Read the model definition and answer for the solid it produces. Units are mm, in the model's axes. A direction names the side the tool comes from. Round coordinates to 2 decimals unless told otherwise and drop trailing zeros. Loops run counter-clockwise (first coordinate to the right, second up) from the corner with the lowest first, then second, coordinate; pieces in that order, holes last. Notation, with made-up numbers: M -31.75,76.5 L -0.75,76.5 A20 ccw -0.75,88.5 Z; hole C 50.25,56 d2. An arc over 180 degrees is marked long. Answer as CSV lines item,"result".
```python
from build123d import *

# Parameters (mm, degrees)
SALIENTE_EXTRUIR1_DEPTH = 3


with BuildPart() as part:
    # Croquis1 → Saliente-Extruir1 (new body)
    with BuildSketch(Plane(origin=(0, 0, 0), x_dir=(1, 0, 0), z_dir=(0, 1, 0))):
        with BuildLine():
            Line((-59, 0), (-17, 0))
            Line((-17, 0), (-14, 0))
            Line((-14, 0), (-14, -7))
            Line((-14, -7), (-11, -7))
            Line((-11, -7), (-11, 0))
            Line((-11, 0), (-4.5, 0))
            ThreePointArc((-4.5, 0), (0, -4.5), (4.5, 0))
            Line((4.5, 0), (11, 0))
            Line((11, 0), (11, -7))
            Line((11, -7), (14, -7))
            Line((14, -7), (14, 0))
            Line((14, 0), (17, 0))
            Line((17, 0), (59, 0))
            Line((59, 0), (59, -20))
            Line((59, -20), (62, -20))
            Line((62, -20), (62, 0))
            Line((62, 0), (70, 0))
            ThreePointArc((70, 0), (0, -70), (-70, 0))
            Line((-70, 0), (-62, 0))
            Line((-62, 0), (-62, -20))
            Line((-62, -20), (-59, -20))
            Line((-59, -20), (-59, 0))
        make_face()
        Polygon((-7, -14), (7, -14), (7, -11), (0, -11), (-7, -11), align=None, mode=Mode.SUBTRACT)
        Polygon((24.748737342, -24.748737342), (17.67766953, -31.819805153), (19.798989873, -33.941125497), (33.941125497, -19.798989873), (31.819805153, -17.67766953), align=None, mode=Mode.SUBTRACT)
        Polygon((-24.748737342, -24.748737342), (-31.819805153, -17.67766953), (-33.941125497, -19.798989873), (-19.798989873, -33.941125497), (-17.67766953, -31.819805153), align=None, mode=Mode.SUBTRACT)
        Polygon((27.577164466, -55.861435714), (55.861435714, -27.577164466), (57.982756057, -29.69848481), (43.840620434, -43.840620434), (29.69848481, -57.982756057), align=None, mode=Mode.SUBTRACT)
        Polygon((-20, -59), (20, -59), (20, -62), (0, -62), (-20, -62), align=None, mode=Mode.SUBTRACT)
        Polygon((-55.861435714, -27.577164466), (-27.577164466, -55.861435714), (-29.69848481, -57.982756057), (-43.840620434, -43.840620434), (-57.982756057, -29.69848481), align=None, mode=Mode.SUBTRACT)
    extrude(amount=SALIENTE_EXTRUIR1_DEPTH)


solid = part.part
```
1) Each of these flat-tipped pins is pushed along its axis until it touches: P1, Ø0.9, axis at y = 1.5, z = 10, coming from the -X side; P2, Ø0.9, axis at y = 1, z = 12.5, coming from the +X side; P3, Ø1.5, axis at y = 2, z = 4.5, coming from the -X side; P4, Ø1.5, axis at x = -4, y = 2, coming from the -Z side. Where does it stop, or does it pass through?
Evaluation:
P1,"stops at x = -69.35"
P2,"stops at x = 68.96"
P3,"stops at x = -69.9"
P4,"stops at z = 0"
2) Find section A-A, the plane x = 0. Give the vertices of the cut face in (y, z), then the cut area to 4 significant figures.
Evaluation:
outline,"M 0,4.5 L 3,4.5 L 3,11 L 0,11 Z; M 0,14 L 3,14 L 3,59 L 0,59 Z; M 0,62 L 3,62 L 3,70 L 0,70 Z"
area,"178.5 mm^2"
3) Find section B-B, the plane z = 52.5. Give the vertices of the cut face in (x, y), then the cut area to 3 significant figures.
Evaluation:
outline,"M -46.3,0 L -35.18,0 L -35.18,3 L -46.3,3 Z; M -30.94,0 L 30.94,0 L 30.94,3 L -30.94,3 Z; M 35.18,0 L 46.3,0 L 46.3,3 L 35.18,3 Z"
area,"252 mm^2"
4) Straight lines are drawn through the part: line 1 (X direction, y = 1.6, z = 46); line 2 (Z direction, x = -18, y = 0.3); line 3 (X direction, y = 1.95, z = 21.5). For each, find the intervals that lie inside material, in ascending order.
Evaluation:
line 1,"x = -52.76 to -41.68, -37.44 to 37.44, 41.68 to 52.76"
line 2,"z = 0 to 31.5, 32.14 to 59, 62 to 67.65"
line 3,"x = -66.62 to -32.24, -28 to 28, 32.24 to 66.62"
5) Find section C-C, the plane x = 48. Give the vertices of the cut face in (y, z), then the cut area to 3 significant figures.
Evaluation:
outline,"M 0,0 L 3,0 L 3,35.44 L 0,35.44 Z; M 0,39.68 L 3,39.68 L 3,50.95 L 0,50.95 Z"
area,"140 mm^2"
6) A tool of negligible diameter and unlimited length cuts with its end or side. For faces 4 (the flat face through (36, 1, 0)), 5 (the flat face through (59, 1, 10)), 6 (the flat face through (-7, 1, 12)), from which of +Z, -Z, +X, -X, +Y, -Y can it reach the whole face along a straight path? Write none if from no direction.
Evaluation:
face 4,"-Z, +X, -X, +Y, -Y"
face 5,"-Z, +Y, -Y"
face 6,"+Y, -Y"
7) Find section D-D, the plane y = 0.5. Count the separate pieces of the cut face and the enclosed holes in it, then the cut area to 3 significant figures.
Evaluation:
separate pieces,"1"
enclosed holes,"6"
area,"6,980 mm^2"
8) Determine the mould class of faces 1 (the flat face through (26.77, 1.48, 26.97)), 2 (the cylindrical face through (1.539, 1.479, 69.983)), 3 (the flat face through (-66, 1, 0)) for opening direction X: released by +X, released by -X, zero draft, split by the parting line, or undercut.
Evaluation:
face 1,"undercut"
face 2,"split by the parting line"
face 3,"zero draft"
